```python
from build123d import *

# Parameters (mm, degrees)
F1_DEPTH = 3
F2_DEPTH = 3
F4_DEPTH = 3


with BuildPart() as f1:
    # F0 (on Top) → F1 (new body)
    with BuildSketch(Plane.XY):
        with BuildLine():
            Line((0, 2.5), (-7.0710678119, 2.5))
            ThreePointArc((-7.0710678119, 2.5), (-7.5, 0), (-7.0710678119, -2.5))
            Line((-7.0710678119, -2.5), (0, -2.5))
            Line((0, -2.5), (0, 0))
            Line((0, 0), (0, 2.5))
        make_face()
        with BuildLine():
            ThreePointArc((-7.0710678119, -2.5), (-4.3301270189, -6.123724357), (0, -7.5))
            Line((0, -7.5), (0, -2.5))
            Line((0, -2.5), (-7.0710678119, -2.5))
        make_face()
        with BuildLine():
            Line((0, 2.5), (0, 7.5))
            ThreePointArc((0, 7.5), (-4.3301270189, 6.123724357), (-7.0710678119, 2.5))
            Line((-7.0710678119, 2.5), (0, 2.5))
        make_face()
    extrude(amount=-F1_DEPTH)

    # F0 (on Top) → F2 (join)
    with BuildSketch(Plane.XY):
        with BuildLine():
            ThreePointArc((-7.0710678119, 2.5), (-4.3301270189, 6.123724357), (0, 7.5))
            Line((0, 7.5), (-10, 7.5))
            Line((-10, 7.5), (-10, 2.5))
            Line((-10, 2.5), (-7.0710678119, 2.5))
        make_face()
        with BuildLine():
            Line((0, 2.5), (0, 7.5))
            ThreePointArc((0, 7.5), (-4.3301270189, 6.123724357), (-7.0710678119, 2.5))
            Line((-7.0710678119, 2.5), (0, 2.5))
        make_face()
        with BuildLine():
            Line((-10, -7.5), (0, -7.5))
            ThreePointArc((0, -7.5), (-4.3301270189, -6.123724357), (-7.0710678119, -2.5))
            Line((-7.0710678119, -2.5), (-10, -2.5))
            Line((-10, -2.5), (-10, -7.5))
        make_face()
        with BuildLine():
            ThreePointArc((-7.0710678119, -2.5), (-4.3301270189, -6.123724357), (0, -7.5))
            Line((0, -7.5), (0, -2.5))
            Line((0, -2.5), (-7.0710678119, -2.5))
        make_face()
    extrude(amount=F2_DEPTH)

    # F3 (on face) → F4 (join)
    with BuildSketch(Plane(origin=(0, 0, -3), x_dir=(1, 0, 0), z_dir=(0, 0, -1))):
        with BuildLine():
            Line((0, -7.5), (0, 7.5))
            ThreePointArc((0, 7.5), (-7.5, 0), (0, -7.5))
        make_face()
        with BuildLine():
            Line((0, 7.5), (0, 8))
            ThreePointArc((0, 8), (-8, 0), (0, -8))
            Line((0, -8), (0, -7.5))
            ThreePointArc((0, -7.5), (-7.5, 0), (0, 7.5))
        make_face()
    extrude(amount=F4_DEPTH)


solid = f1.part
```
Can you work these out from the model? Positions are in its coordinate system, mm. A direction names the side the tool comes from. Coordinates: 2 decimals unless noted, no trailing zeros. Loops run counter-clockwise (first coordinate to the right, second up) from the corner with the lowest first, then second, coordinate; pieces in that order, holes last.
Item 1: If we mould it in two halves opening along Y, with no side actions, what happens to faces 1 (the face through (-8, 0, -4)), 2 (the face through (-5, -2.5, 1)), 3 (the face through (-3, 0, -6))? For each: released by +Y, released by -Y, zero draft, split by the parting line, or undercut.
Answers below:
face 1: split by the parting line
face 2: undercut
face 3: zero draft
Item 2: Suppose I cut it at A-A (x = -8.75). Please give me the cut outline in (y, z).
Answers below:
outline: (-7.5, 0) - (-2.5, 0) - (-2.5, 3) - (-7.5, 3) - close; (2.5, 0) - (7.5, 0) - (7.5, 3) - (2.5, 3) - close
Item 3: Suppose I cut it at B-B (z = 1). Please give me the cut outline in (x, y), then the cut area to 3 significant figures.
Answers below:
outline: (-10, -7.5) - (0, -7.5) - (0, -2.5) - (-10, -2.5) - close; (-10, 2.5) - (0, 2.5) - (0, 7.5) - (-10, 7.5) - close
area: 100 mm2
Item 4: Suppose I cut it at D-D (x = -5.75). Please give me the cut outline in (y, z).
Answers below:
outline: (-7.5, 0) - (-4.82, 0) - (-4.82, -3) - (-5.56, -3) - (-5.56, -6) - (5.56, -6) - (5.56, -3) - (4.82, -3) - (4.82, 0) - (7.5, 0) - (7.5, 3) - (2.5, 3) - (2.5, 0) - (-2.5, 0) - (-2.5, 3) - (-7.5, 3) - close
Item 5: Which directions (+Z, -Z, +X, -X, +Y, -Y) give clear straight access to the entire face, cutting with the end or side of a thin tool? Please do faces 4 (the face through (-5, 7.5, 1)), 5 (the face through (-7, -6, 0)), 6 (the face through (-5, 2.5, 1)), 7 (the face through (-7, 6, 0)).
Answers below:
face 4: +Z, +X, -X, +Y
face 5: -X, -Y
face 6: +Z, +X, -X
face 7: -X, +Y
Item 6: I'm going to push flat-ended pins straight in: pin 1 (2.5 mm diameter, centred on x = -4, z = 1, fed in from -Y); pin 2 (3.5 mm diameter, centred on x = -4, z = 2, fed in from +Y); pin 3 (1 mm diameter, centred on x = -7.5, y = -4.5, fed in from -Z). Where does each tip first touch, or does it pass through?
Answers below:
pin 1: stops at y = -7.5
pin 2: stops at y = 7.5
pin 3: stops at z = 0
Item 7: Suppose I cut it at C-C (y = 6). Please give me the cut outline in (x, z).
Answers below:
outline: (-10, 0) - (-4.5, 0) - (-4.5, -3) - (-5.29, -3) - (-5.29, -6) - (0, -6) - (0, 3) - (-10, 3) - close
Item 8: Please list where these lines run through material, in increasing order: L1, parallel to Y at x = -1.5, z = 1.5; L2, parallel to Z at x = -8.5, y = 3.25; L3, parallel to Z at x = -3.25, y = 1.5.
Answers below:
L1: y = -7.5 to -2.5, 2.5 to 7.5
L2: z = 0 to 3
L3: z = -6 to 0
